Work out the finished part from the listing and answer in its coordinate system (mm). A direction names the side the tool comes from. Coordinates: 2 decimals unless noted, no trailing zeros. Write each loop counter-clockwise with the first axis right and the second up, starting at its lowest first coordinate (ties: lowest second). Pieces come first, ordered by that corner, then holes. Notation, with made-up numbers: (64.5, 15.5) - (71.5, 15.5) arc R17 ccw to (71.5, 43.5) - close; hole circle Ø9 at (42, 25.25). An arc over 180 degrees is marked (long way). Use a Markdown table: item, result. Add a question column.
(1) The part is cut by section D-D, the plane z = 33. Give the vertices of the cut face in (x, y) (3 decimals).
(2) Given pin 1 Ø10.5 at (x, y) = (-3.5, -3.5) entering from +Z; pin 2 Ø1 at (x, y) = (7, -1) entering from -Z; pin 3 Ø2.5 at (x, z) = (0, 37.5) entering from -Y, each flat-ended and moving along its own axis, determine where each tip first touches the part or whether it passes through.
(3) For a pull along Z with two mould halves and no side action, classify faces 1 (the face through (0, -11, 0)), 2 (the face through (0.986, -16.968, 38.786)), 3 (the face through (5, 1, 19.5)), 4 (the face through (15, -6, 25)) as released by +Z, released by -Z, zero draft, split by the parting line, or undercut.
(4) The part is cut by section B-B, the plane y = -3.62. Give the vertices of the cut face in (x, z) (3 decimals).
(5) The part is cut by section A-A, the plane z = 4.5. Give the vertices of the cut face in (x, y).
(6) Find the intervals of material crossed by line 1 (Z direction, x = 0, y = -15.8); line 2 (X direction, y = -17.65, z = 37.5); line 3 (Y direction, x = 0, z = 34.5) (3 decimals), in increasing order. Write a range as from..to.
(7) A tool of negligible diameter and unlimited length cuts with its end or side. For faces 5 (the face through (-3.16, -13.66, 34.54)), 6 (the face through (14, 9, 25)), 7 (the face through (1.582, -16.958, 12.851)), from which of +Z, -Z, +X, -X, +Y, -Y can it reach the whole face along a straight path? Write none if from no direction.
(8) The part is cut by section C-C, the plane x = 4.75. Give the vertices of the cut face in (y, z).
Autodesk Inventor part; units mm, degrees
ref_plane "YZ Plane" through (0, 0, 0) normal (1, 0, 0) x (0, 1, 0)
ref_plane "XZ Plane" through (0, 0, 0) normal (0, 1, 0) x (-1, 0, 0)
ref_plane "XY Plane" through (0, 0, 0) normal (0, 0, 1) x (1, 0, 0)
sketch "Esboço2" plane through (0, 0, 0) normal (0, 0, 1) x (1, 0, 0)
  line L0 (-15, 10) -> (15, 10)
  line L1 (15, 10) -> (15, -20)
  line L2 (15, -20) -> (-15, -20)
  line L3 (-15, -20) -> (-15, 10)
  line L4 (-15, 10) -> (15, -20) construction
  line L5 (15, 10) -> (-15, -20) construction
  point P0 (0, -5)
  dimension "d10" = 30
  dimension "d11" = 30
extrude "Extrusão1" add sketch "Esboço2" along normal blind 50
sketch "Esboço3" plane through (0, 0, 50) normal (0, 0, 1) x (1, 0, 0)
  line L0 (15, 10) -> (-15, 10)
  line L1 (0, 10) -> (0, -3.62)
  circle A0 centre (0, -3.62) radius 10.5
  point P0 (0, 0)
  dimension "d14" = 13.62
  dimension "d15" = 21
hole "Furo1" at (0, -3.62, 50) direction (0, 0, -1) diameter 13 end through all counterbore diameter 21.05 counterbore depth 30.5
sketch "Esboço4" plane through (-15, -20, 0) normal (0, -1, 0) x (1, 0, 0)
  line L0 (15, 0) -> (15, 50)
  line L1 (30, 50) -> (0, 50)
  circle A0 centre (15, 12.5) radius 1.6056 construction
  circle A1 centre (15, 37.5) radius 1.4692 construction
  line L2 (0, 0) -> (0, 50) construction
  line L3 (0, 25) -> (30, 25) construction
  line L4 (30, 0) -> (30, 50) construction
  dimension "d23" = 12.5
  dimension "d24" = 12.5
hole "Furo2" at (0, -20, 12.5) at (0, -20, 37.5) direction (0, 1, 0) diameter 3.242 depth 6 tip angle 118
chamfer "Chanfro1" distance 2 angle 45 2 edges at (15, 10, 25) (-15, 10, 25)
properties part number "blocoSuporteRolamentos"
Model answer:
| question | item | result |
|---|---|---|
| 1 | outline | (-15, -20) - (15, -20) - (15, 8) - (13, 10) - (-13, 10) - (-15, 8) - close; hole circle Ø21.05 at (0, -3.62) |
| 2 | pin 1 | z = 19.5 |
| 2 | pin 2 | z = 0 |
| 2 | pin 3 | y = 6.83 |
| 3 | face 1 | released by -Z |
| 3 | face 2 | undercut |
| 3 | face 3 | released by +Z |
| 3 | face 4 | zero draft |
| 4 | outline | (-15, 0) - (-6.5, 0) - (-6.5, 19.5) - (-10.525, 19.5) - (-10.525, 50) - (-15, 50) - close; (6.5, 0) - (15, 0) - (15, 50) - (10.525, 50) - (10.525, 19.5) - (6.5, 19.5) - close |
| 5 | outline | (-15, -20) - (15, -20) - (15, 8) - (13, 10) - (-13, 10) - (-15, 8) - close; hole circle Ø13 at (0, -3.62) |
| 6 | line 1 | 0..10.88, 14.12..35.88, 39.12..50 |
| 6 | line 2 | -15..-1.62, 1.62..15 |
| 6 | line 3 | -20..-14.145, 6.905..10 |
| 7 | face 5 | +Z |
| 7 | face 6 | +Z, -Z, +X, +Y |
| 7 | face 7 | -Y |
| 8 | outline | (-20, 0) - (-8.06, 0) - (-8.06, 19.5) - (-13.01, 19.5) - (-13.01, 50) - (-20, 50) - close; (0.82, 0) - (10, 0) - (10, 50) - (5.77, 50) - (5.77, 19.5) - (0.82, 19.5) - close |
